Geometry: final body of the model. Coordinates: model frame, mm. A direction names the side the tool comes from. Give positions to 0.01 mm unless a question says otherwise; leave off trailing zeros. Write each loop counter-clockwise with the first axis right and the second up, starting at its lowest first coordinate (ties: lowest second). Pieces come first, ordered by that corner, then holes. Notation, with made-up numbers: (50, -25) -> (77, -25) arc R25 cw to (77, -9) -> close; hole circle Ø1 at (-26, -3.75). An arc over 180 degrees is marked (long way). Answer as a JSON object with one key per item and string values.
from build123d import *

# Parameters (mm, degrees)
SKETCH1_R                 = 7
BOSS_EXTRUDE1_DEPTH       = 15
F_8_0MM_DOWEL_HOLE1_D     = 8
F_8_0MM_DOWEL_HOLE1_DEPTH = 30
F_8_0MM_DOWEL_HOLE1_TIP   = 2.403442476
SKETCH3_R                 = 7
SKETCH3_R_2               = 4
BOSS_EXTRUDE2_DEPTH       = 15


with BuildPart() as part:
    # Sketch1 → Boss-Extrude1 (new body)
    with BuildSketch(Plane.XY):
        with BuildLine():
            Line((-10, 0), (10, 0))
            Line((10, 0), (10, 8))
            Line((10, 8), (25, 8))
            Line((25, 8), (17, 93))
            ThreePointArc((17, 93), (0, 110), (-17, 93))
            Line((-17, 93), (-25, 8))
            Line((-25, 8), (-10, 8))
            Line((-10, 8), (-10, 0))
        make_face()
        with Locations((0, 93)):
            Circle(SKETCH1_R, mode=Mode.SUBTRACT)
    extrude(amount=BOSS_EXTRUDE1_DEPTH)

    # Ø8.0mm Dowel Hole1
    with Locations(Plane(origin=(0, 0, 7.5), x_dir=(0, 0, -1), z_dir=(0, -1, 0))):
        with Locations((0, 0)):
            Hole(F_8_0MM_DOWEL_HOLE1_D / 2, depth=F_8_0MM_DOWEL_HOLE1_DEPTH)
            with Locations((0, 0, -(F_8_0MM_DOWEL_HOLE1_DEPTH + F_8_0MM_DOWEL_HOLE1_TIP / 2))):  # 118° drill point
                Cone(0, F_8_0MM_DOWEL_HOLE1_D / 2, F_8_0MM_DOWEL_HOLE1_TIP, mode=Mode.SUBTRACT)

    # Sketch3 → Boss-Extrude2 (add, through all)
    with BuildSketch(Plane.XY.offset(15)):
        with Locations((0, 93)):
            Circle(SKETCH3_R)
        with Locations((0, 93)):
            Circle(SKETCH3_R_2, mode=Mode.SUBTRACT)
    extrude(amount=-BOSS_EXTRUDE2_DEPTH)


solid = part.part
Q1. Cut plane A-A (z = 12.5). Return the cut outline in (x, y), and give its area (3 significant figures).
Values:
{"outline": "(-25, 8) -> (-10, 8) -> (-10, 0) -> (10, 0) -> (10, 8) -> (25, 8) -> (17, 93) arc R17 ccw to (-17, 93) -> close; hole circle Ø8 at (0, 93)", "area": "4,130 mm²"}
Q2. Cut plane D-D (x = 19.5). Return the cut outline in (y, z).
Values:
{"outline": "(8, 0) -> (66.44, 0) -> (66.44, 15) -> (8, 15) -> close"}
Q3. First-contact query: P1, Ø1, axis at y = 89.5, z = 3.5, coming from the -X side; P2, Ø1.5, axis at y = 65, z = 5, coming from the +X side; P3, Ø2, axis at x = 13, z = 5, coming from the -Y side. Flat tips, straight axial feed; report the tip coordinate or a pass-through.
Values:
{"P1": "x = -17.38", "P2": "x = 19.71", "P3": "y = 8"}
Q4. Cut plane C-C (y = 50.5). Return the cut outline in (x, z).
Values:
{"outline": "(-21, 0) -> (21, 0) -> (21, 15) -> (-21, 15) -> close"}
Q5. Set-up query: faces 5 (the flat face through (-2.4, 0, 4.1)), 6 (the flat face through (10, 4, 7)), 7 (the flat face through (-10, 4, 7)). Return all of +Z, -Z, +X, -X, +Y, -Y with unobstructed straight access to the full face (end or side cutting, diameter ignored); none if empty.
Values:
{"face 5": "+Z, -Z, +X, -X, -Y", "face 6": "+Z, -Z, +X, -Y", "face 7": "+Z, -Z, -X, -Y"}
Q6. Material intervals for L1, parallel to Z at x = 0, y = 7; L2, parallel to Y at x = 2.5, z = 9.75; L3, parallel to Z at x = 1.5, y = 23, sorted ascending. Write a range as from..to.
Values:
{"L1": "0..3.5, 11.5..15", "L2": "30.38..89.88, 96.12..109.82", "L3": "0..3.79, 11.21..15"}
Q7. Mould query, pull axis Z, two halves, no side actions, for faces 1 (the flat face through (0, 56, 0)), 2 (the cylindrical face through (1.846, 89.451, 7.605)), 3 (the conical face through (-0.423, 31.986, 8.051)), 4 (the cylindrical face through (-2.4, 15.2, 4.3)). Classes: pulls with the +Z half, pulls with the -Z half, needs draft (parallel to the pull), parting line crosses it, or undercut.
Values:
{"face 1": "pulls with the -Z half", "face 2": "needs draft", "face 3": "undercut", "face 4": "undercut"}
Q8. Cut plane B-B (y = 29). Return the cut outline in (x, z), and give its area (3 significant figures).
Values:
{"outline": "(-23.02, 0) -> (23.02, 0) -> (23.02, 15) -> (-23.02, 15) -> close; hole circle Ø8 at (0, 7.5)", "area": "640 mm²"}
